Here's how the part is built. I have some questions about the finished solid (model axes, mm). Face numbers are marked on the shaded views. A direction names the side the tool comes from. Coordinates: 2 decimals unless noted, no trailing zeros. Write each loop counter-clockwise with the first axis right and the second up, starting at its lowest first coordinate (ties: lowest second). Pieces come first, ordered by that corner, then holes.
(1) Imagine slicing it at D-D, the plane x = 29.5. List the corners of the cut face in (y, z) for me.
(2) Imagine slicing it at A-A, the plane y = 40.5. List the corners of the cut face in (x, z) for me, plus the area to 3 significant figures.
(3) Imagine slicing it at C-C, the plane z = 14.5. List the corners of the cut face in (x, y) for me, plus the area to 3 significant figures.
(4) Thinking about a two-plate mould opening in Y: for the marked faces 1, 2, 3 and 4, which applies, released by +Y, released by -Y, zero draft, split by the parting line, or undercut?
(5) Please list where these lines run through material, in increasing order: probe 1 along Z at (x, y) = (5.5, 31.75); probe 2 along Z at (x, y) = (5, 31); probe 3 along X at (y, z) = (42, 21).
(6) Imagine slicing it at B-B, the plane y = 31.75. List the corners of the cut face in (x, z) for me, plus the area to 3 significant figures.
(7) For pin 1 Ø10.5 at (x, y) = (44.5, 24.5) entering from +Z; pin 2 Ø1.5 at (x, y) = (80.5, 10) entering from -Z; pin 3 Ø2 at (y, z) = (28, 33) entering from -X, each with a flat end and sliding along its axis, tell me the tip position at first contact or that it passes through.
(8) Which directions (+Z, -Z, +X, -X, +Y, -Y) give clear straight access to the entire face, cutting with the end or side of a thin tool? Please do the marked faces 5, 6 and 7.
```python
from build123d import *

# Parameters (mm, degrees)
F0_W      = 84.074
F0_H      = 76.2
F1_DEPTH  = 63.5
F2_W      = 66.548
F2_H      = 68.326
F3_DEPTH  = 63.501
F5_DEPTH  = 25.4
F4_W      = 14.478
F4_H      = 7.874
F6_DEPTH  = 84.075
F4_R      = 7.112
F7_DEPTH  = 25.4
F9_DEPTH  = 84.075
F10_DEPTH = 25.4


with BuildPart() as f1:
    # F0 (on Front) → F1 (new body)
    with BuildSketch(Plane.XZ):
        with Locations((42.037, 38.1)):
            Rectangle(F0_W, F0_H)
    extrude(amount=-F1_DEPTH)

    # F2 (on face) → F3 (cut, through all)
    with BuildSketch(Plane.XZ):
        with Locations((41.148, 42.037)):
            Rectangle(F2_W, F2_H)
    extrude(amount=-F3_DEPTH, mode=Mode.SUBTRACT)

    # F4 (on face) → F5 (cut)
    with BuildSketch(Plane(origin=(0, 0, 0), x_dir=(0, -1, 0), z_dir=(-1, 0, 0))):
        with BuildLine():
            Line((-63.5, 7.874), (-49.022, 7.874))
            Line((-49.022, 7.874), (-49.022, 55.626))
            ThreePointArc((-49.022, 55.626), (-31.75, 72.898), (-14.478, 55.626))
            Line((-14.478, 55.626), (-14.478, 7.874))
            Line((-14.478, 7.874), (0, 7.874))
            Line((0, 7.874), (0, 76.2))
            Line((0, 76.2), (-63.5, 76.2))
            Line((-63.5, 76.2), (-63.5, 7.874))
        make_face()
    extrude(amount=-F5_DEPTH, mode=Mode.SUBTRACT)

    # F4 (on face) → F6 (cut, through all)
    with BuildSketch(Plane(origin=(0, 0, 0), x_dir=(0, -1, 0), z_dir=(-1, 0, 0))):
        with Locations((-56.261, 3.937)):
            Rectangle(F4_W, F4_H)
        with Locations((-7.239, 3.937)):
            Rectangle(F4_W, F4_H)
    extrude(amount=-F6_DEPTH, mode=Mode.SUBTRACT)

    # F4 (on face) → F7 (cut)
    with BuildSketch(Plane(origin=(0, 0, 0), x_dir=(0, -1, 0), z_dir=(-1, 0, 0))):
        with Locations((-31.75, 36.576)):
            Circle(F4_R)
        with Locations((-31.75, 55.626)):
            Circle(F4_R)
    extrude(amount=-F7_DEPTH, mode=Mode.SUBTRACT)

    # F8 (on face) → F9 (cut, through all)
    with BuildSketch(Plane.YZ.offset(84.074)):
        with BuildLine():
            Line((0, 7.874), (14.478, 7.874))
            Line((14.478, 7.874), (14.478, 45.974))
            ThreePointArc((14.478, 45.974), (13.840888, 47.512124), (12.302764, 48.149236))
            Line((12.302764, 48.149236), (9.398, 48.149236))
            ThreePointArc((9.398, 48.149236), (1.921236, 55.626), (9.398, 63.102764))
            Line((9.398, 63.102764), (31.75, 63.102764))
            Line((31.75, 63.102764), (54.102, 63.102764))
            ThreePointArc((54.102, 63.102764), (61.578764, 55.626), (54.102, 48.149236))
            Line((54.102, 48.149236), (51.197236, 48.149236))
            ThreePointArc((51.197236, 48.149236), (49.659112, 47.512124), (49.022, 45.974))
            Line((49.022, 45.974), (49.022, 7.874))
            Line((49.022, 7.874), (63.5, 7.874))
            Line((63.5, 7.874), (63.5, 76.2))
            Line((63.5, 76.2), (0, 76.2))
            Line((0, 76.2), (0, 7.874))
        make_face()
    extrude(amount=-F9_DEPTH, mode=Mode.SUBTRACT)

    # F8 (on face) → F10 (cut)
    with BuildSketch(Plane.YZ.offset(84.074)):
        with BuildLine():
            ThreePointArc((54.102, 52.07), (57.658, 55.626), (54.102, 59.182))
            Line((54.102, 59.182), (31.75, 59.182))
            Line((31.75, 59.182), (9.398, 59.182))
            ThreePointArc((9.398, 59.182), (5.842, 55.626), (9.398, 52.07))
            Line((9.398, 52.07), (31.75, 52.07))
            Line((31.75, 52.07), (54.102, 52.07))
        make_face()
    extrude(amount=-F10_DEPTH, mode=Mode.SUBTRACT)


solid = f1.part
```
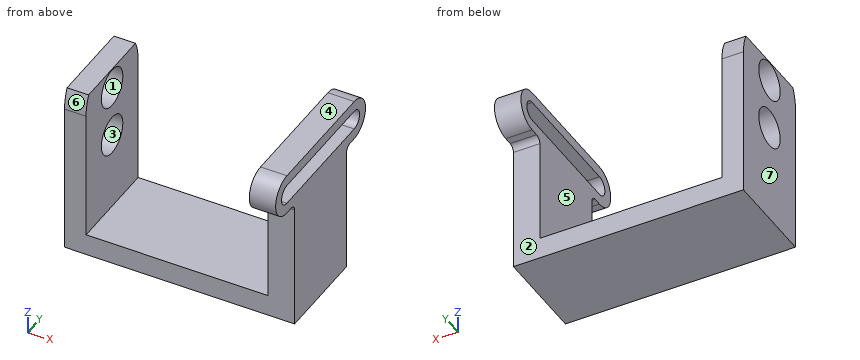
Recorded:
1. outline: (14.48, 0) - (49.02, 0) - (49.02, 7.87) - (14.48, 7.87) - close
2. outline: (0, 0) - (84.07, 0) - (84.07, 52.07) - (74.42, 52.07) - (74.42, 7.87) - (7.87, 7.87) - (7.87, 63.1) - (0, 63.1) - close; (74.42, 59.18) - (84.07, 59.18) - (84.07, 63.1) - (74.42, 63.1) - close
2. area: 1,560 mm2
3. outline: (0, 14.48) - (7.87, 14.48) - (7.87, 49.02) - (0, 49.02) - close; (74.42, 14.48) - (84.07, 14.48) - (84.07, 49.02) - (74.42, 49.02) - close
3. area: 605 mm2
4. face 1: undercut
4. face 2: released by +Y
4. face 3: undercut
4. face 4: zero draft
5. probe 1: z = 0 to 29.46, 43.69 to 48.51, 62.74 to 63.1
5. probe 2: z = 0 to 29.5, 43.65 to 48.55, 62.7 to 63.1
5. probe 3: x = 0 to 7.87, 74.42 to 84.07
6. outline: (0, 0) - (84.07, 0) - (84.07, 52.07) - (74.42, 52.07) - (74.42, 7.87) - (7.87, 7.87) - (7.87, 29.46) - (0, 29.46) - close; (0, 43.69) - (7.87, 43.69) - (7.87, 48.51) - (0, 48.51) - close; (0, 62.74) - (7.87, 62.74) - (7.87, 63.1) - (0, 63.1) - close; (74.42, 59.18) - (84.07, 59.18) - (84.07, 63.1) - (74.42, 63.1) - close
6. area: 1,340 mm2
7. pin 1: stops at z = 7.87
7. pin 2: stops at z = 48.15
7. pin 3: stops at x = 74.42
8. face 5: +Z, +Y, -Y
8. face 6: +Z, -X, -Y
8. face 7: +Z, -Z, -X, +Y, -Y
